Can you work these out from the model? Positions are in its coordinate system, mm. Give positions to 0.01 mm unless a question says otherwise; leave off trailing zeros. Order: outer loops, then holes, each group sorted by start corner. A loop starts at its lowest first (then second) coordinate and runs counter-clockwise, first axis right, second up.
Item 1: If we mould it in two halves opening along X, with no side actions, what happens to faces 1 (the cylindrical face through (48.81, 52.56, 5.07)), 2 (the flat face through (10, 80, 5)), 3 (the flat face through (0, 39, 5)), 4 (the cylindrical face through (9.7, 52, 5.1))? For each: +X half, -X half, draft (parallel to the pull), parting line (faces both ways), or undercut.
Item 2: I want a section at D-D, the plane x = 50. Write out the boundary of the cut face in (y, z), then the cut area to 3 significant figures.
Item 3: If I drill on line 1 along Y through (x, z) = (10, 7.75); line 2 along Y through (x, z) = (50, 4.25); line 3 along X through (y, z) = (31, 6.5), over which ranges is the centre line in solid material (lowest first)?
Item 4: I'm going to push flat-ended pins straight in: pin 1 Ø2.5 at (x, y) = (10, 53.47) entering from -Z; pin 2 Ø1 at (y, z) = (41, 4) entering from +X; pin 3 Ø2 at (y, z) = (14.5, 3) entering from +X; pin 4 Ø6 at (y, z) = (38, 7.5) entering from +X. Where does each tip first touch, or does it pass through?
Item 5: I want a section at C-C, the plane y = 53.47. Write out the boundary of the cut face in (x, z).
Item 6: I want a section at A-A, the plane x = 10. Write out the boundary of the cut face in (y, z).
Item 7: I want a section at B-B, the plane z = 2.5. Write out the boundary of the cut face in (x, y), then the cut area to 3 significant figures.
```python
from build123d import *

# Parameters (mm, degrees)
PAD_DEPTH    = 10
SKETCH001_R  = 1.5
POCKET_DEPTH = 10.001


with BuildPart() as part:
    # Sketch → Pad (new body)
    with BuildSketch(Plane.XY):
        with BuildLine():
            Line((0, 0), (140, 0))
            ThreePointArc((140, 0), (139.04534, 4.264014), (136.363636, 7.713892))
            Line((70.909026, 61.711191), (136.363636, 7.713892))
            ThreePointArc((70.909026, 61.711191), (47.047216, 75.289097), (19.999983, 80))
            Line((0, 80), (19.999983, 80))
            Line((0, 0), (0, 80))
        make_face()
    extrude(amount=PAD_DEPTH)

    # Sketch001 → Pocket (cut, through all)
    with BuildSketch(Plane.XY.offset(10)):
        with Locations((10, 53.47)):
            Circle(SKETCH001_R)
        with Locations((50, 53.47)):
            Circle(SKETCH001_R)
    extrude(amount=-POCKET_DEPTH, mode=Mode.SUBTRACT)


solid = part.part
```
Results list:
1. face 1: undercut
1. face 2: draft
1. face 3: -X half
1. face 4: undercut
2. outline: (0, 0) - (51.97, 0) - (51.97, 10) - (0, 10) - close; (54.97, 0) - (74.16, 0) - (74.16, 10) - (54.97, 10) - close
2. area: 712 mm2
3. line 1: y = 0 to 51.97, 54.97 to 80
3. line 2: y = 0 to 51.97, 54.97 to 74.16
3. line 3: x = 0 to 108.14
4. pin 1: passes through
4. pin 2: stops at x = 96.62
4. pin 3: stops at x = 129.35
4. pin 4: stops at x = 103.29
5. outline: (0, 0) - (8.5, 0) - (8.5, 10) - (0, 10) - close; (11.5, 0) - (48.5, 0) - (48.5, 10) - (11.5, 10) - close; (51.5, 0) - (80.9, 0) - (80.9, 10) - (51.5, 10) - close
6. outline: (0, 0) - (51.97, 0) - (51.97, 10) - (0, 10) - close; (54.97, 0) - (80, 0) - (80, 10) - (54.97, 10) - close
7. outline: (0, 0) - (140, 0) arc R10 ccw to (136.36, 7.71) - (70.91, 61.71) arc R80 ccw to (20, 80) - (0, 80) - close; hole circle Ø3 at (10, 53.47); hole circle Ø3 at (50, 53.47)
7. area: 7,660 mm2
